The model under review builds one solid part; all positions refer to its coordinate system, in mm. A direction names the side the tool comes from. Round coordinates to 2 decimals unless told otherwise and drop trailing zeros. Write each loop counter-clockwise with the first axis right and the second up, starting at its lowest first coordinate (ties: lowest second). Pieces come first, ordered by that corner, then holes. Notation, with made-up numbers: (-20, -19.5) - (-15, -19.5) arc R28 cw to (-15, -0.5) - close; hole circle Ø3 at (-12, -0.75). An arc over 180 degrees is marked (long way). Write each question's results on one line, items separated by ' | '.
```python
from build123d import *

# Parameters (mm, degrees)
AUFSATZ_LINEAR_AUSTRAGEN1_DEPTH = 145.2
AUFSATZ_LINEAR_AUSTRAGEN2_DEPTH = 145.2
SKIZZE5_R                       = 2.2
SCHNITT_LINEAR_AUSTRAGEN1_DEPTH = 165.848511541
SCHNITT_LINEAR_AUSTRAGEN2_REACH = 166.605
SKIZZE6_W                       = 76.784770152
SKIZZE6_H                       = 124
SKIZZE6_H_2                     = 2.6
SKIZZE7_W                       = 40
SKIZZE7_H                       = 50.4
SCHNITT_LINEAR_AUSTRAGEN3_DEPTH = 166.115329215
SKIZZE8_W                       = 42
SKIZZE8_H                       = 57.4
SCHNITT_LINEAR_AUSTRAGEN4_DEPTH = 3.4


with BuildPart() as part:
    # Skizze1 → Aufsatz-Linear austragen1 (new body)
    with BuildSketch(Plane.XY):
        Polygon((0, 0), (0, 4.329568801), (68.182309499, -23.912468507), (68.182309499, -28.242037309), align=None)
    extrude(amount=AUFSATZ_LINEAR_AUSTRAGEN1_DEPTH)

    # Skizze4 → Aufsatz-Linear austragen2 (add)
    with BuildSketch(Plane.XY.offset(145.2)):
        Polygon((0, 0), (10, -4.142135624), (10, -14.966057627), (0, -10.823922003), align=None)
        Polygon((55.582309499, -23.022946423), (65.582309499, -27.165082046), (65.582309499, -37.989004049), (55.582309499, -33.846868426), align=None)
    extrude(amount=-AUFSATZ_LINEAR_AUSTRAGEN2_DEPTH)

    # Skizze5 → Schnitt-Linear austragen1 (cut, through all)
    with BuildSketch(Plane.XY.offset(145.2)):
        with Locations((5, -7.483028813)):
            Circle(SKIZZE5_R)
        with Locations((60.582309499, -30.505975236)):
            Circle(SKIZZE5_R)
    extrude(amount=-SCHNITT_LINEAR_AUSTRAGEN1_DEPTH, mode=Mode.SUBTRACT)

    # Schnitt-Linear austragen2: up to this face of the body (flat: up to its plane)
    schnitt_linear_austragen2_end = Plane(part.part.faces().sort_by_distance((32.79115475, -13.582541023, 72.6))[0])
    # Skizze6 → Schnitt-Linear austragen2 (cut, up to the picked face)
    with BuildSketch(Plane(origin=(-3.826834324, -9.238795325, 0), x_dir=(0.9238795325112881, -0.3826834323650869, 0), z_dir=(-0.3826834323650869, -0.9238795325112881, 0)), mode=Mode.PRIVATE) as schnitt_linear_austragen2_sk1:
        with Locations((36.735530827, 72.6)):
            Rectangle(SKIZZE6_W, SKIZZE6_H)
    schnitt_linear_austragen2_tool1 = split(extrude(schnitt_linear_austragen2_sk1.sketch, amount=-SCHNITT_LINEAR_AUSTRAGEN2_REACH, mode=Mode.PRIVATE), bisect_by=schnitt_linear_austragen2_end, keep=Keep.BOTH, mode=Mode.PRIVATE)
    # Skizze6 → Schnitt-Linear austragen2 (cut, up to the picked face)
    with BuildSketch(Plane(origin=(-3.826834324, -9.238795325, 0), x_dir=(0.9238795325112881, -0.3826834323650869, 0), z_dir=(-0.3826834323650869, -0.9238795325112881, 0)), mode=Mode.PRIVATE) as schnitt_linear_austragen2_sk2:
        with Locations((36.735530827, 143.9)):
            Rectangle(SKIZZE6_W, SKIZZE6_H_2)
    schnitt_linear_austragen2_tool2 = split(extrude(schnitt_linear_austragen2_sk2.sketch, amount=-SCHNITT_LINEAR_AUSTRAGEN2_REACH, mode=Mode.PRIVATE), bisect_by=schnitt_linear_austragen2_end, keep=Keep.BOTH, mode=Mode.PRIVATE)
    # Skizze6 → Schnitt-Linear austragen2 (cut, up to the picked face)
    with BuildSketch(Plane(origin=(-3.826834324, -9.238795325, 0), x_dir=(0.9238795325112881, -0.3826834323650869, 0), z_dir=(-0.3826834323650869, -0.9238795325112881, 0)), mode=Mode.PRIVATE) as schnitt_linear_austragen2_sk3:
        with Locations((36.735530827, 1.3)):
            Rectangle(SKIZZE6_W, SKIZZE6_H_2)
    schnitt_linear_austragen2_tool3 = split(extrude(schnitt_linear_austragen2_sk3.sketch, amount=-SCHNITT_LINEAR_AUSTRAGEN2_REACH, mode=Mode.PRIVATE), bisect_by=schnitt_linear_austragen2_end, keep=Keep.BOTH, mode=Mode.PRIVATE)
    add(schnitt_linear_austragen2_tool1.solids().sort_by(Axis((30.112371, -23.296874, 72.6), (0.3826834323650869, 0.9238795325112881, 0)))[0], mode=Mode.SUBTRACT)
    add(schnitt_linear_austragen2_tool2.solids().sort_by(Axis((30.112371, -23.296874, 143.9), (0.3826834323650869, 0.9238795325112881, 0)))[0], mode=Mode.SUBTRACT)
    add(schnitt_linear_austragen2_tool3.solids().sort_by(Axis((30.112371, -23.296874, 1.3), (0.3826834323650869, 0.9238795325112881, 0)))[0], mode=Mode.SUBTRACT)

    # Skizze7 → Schnitt-Linear austragen3 (cut, through all)
    with BuildSketch(Plane(origin=(1.530733729, 3.69551813, 0), x_dir=(0.9238795325112881, -0.38268343236508656, 0), z_dir=(0.38268343236508656, 0.9238795325112881, 0))):
        with Locations((35.243145751, -72.6)):
            Rectangle(SKIZZE7_W, SKIZZE7_H)
    extrude(amount=-SCHNITT_LINEAR_AUSTRAGEN3_DEPTH, mode=Mode.SUBTRACT)

    # Skizze8 → Schnitt-Linear austragen4 (cut)
    with BuildSketch(Plane(origin=(0, 0, 0), x_dir=(0.923879532511288, -0.38268343236508684, 0), z_dir=(-0.38268343236508684, -0.923879532511288, 0))):
        with Locations((35.243145751, 75.1)):
            Rectangle(SKIZZE8_W, SKIZZE8_H)
    extrude(amount=-SCHNITT_LINEAR_AUSTRAGEN4_DEPTH, mode=Mode.SUBTRACT)


solid = part.part
```
Q1. We need section B-B (x = 5). State the section outline as (y, z) points.
Evaluation:
outline: (-12.89, 2.6) - (-9.68, 2.6) - (-9.68, 10.6) - (-12.89, 10.6) - close; (-12.89, 134.6) - (-9.68, 134.6) - (-9.68, 142.6) - (-12.89, 142.6) - close; (-5.28, 2.6) - (-2.07, 2.6) - (-2.07, 0) - (2.26, 0) - (2.26, 145.2) - (-2.07, 145.2) - (-2.07, 142.6) - (-5.28, 142.6) - (-5.28, 134.6) - (-2.07, 134.6) - (-2.07, 10.6) - (-5.28, 10.6) - close
Q2. Tool access review of faces 1 (the flat face through (52.603, -19.975, 74.698)), 2 (the flat face through (4, -10, 142.6)), 3 (the flat face through (55.582, -29, 139)), 4 (the flat face through (10, -9, 7)): name each direction out of +Z, -Z, +X, -X, +Y, -Y from which nothing blocks a thin tool from reaching the whole face with its end or side.
Evaluation:
face 1: -X | face 2: +Z, -X, -Y | face 3: +Z, -Z, -X, -Y | face 4: +Z, -Z, -Y
Q3. We need section C-C (z = 20.5). State the section outline as (x, y) points.
Evaluation:
outline: (0, 0) - (68.18, -28.24) - (68.18, -23.91) - (0, 4.33) - close
Q4. For probe 1 along Z at (x, y) = (57.5, -34); probe 2 along Z at (x, y) = (15, -3.5); probe 3 along Y at (x, z) = (5, 7), list the stretches that pass through material, from the lowest coordinate up.
Evaluation:
probe 1: z = 2.6 to 10.6, 134.6 to 142.6 | probe 2: z = 0 to 46.4, 103.8 to 145.2 | probe 3: y = -12.89 to -9.68, -5.28 to 2.26
Q5. Insertion check: P1, Ø5, axis at x = 57.5, z = 90, coming from the +Y side; P2, Ø5, axis at x = 4.5, y = -6.5, coming from the -Z side; P3, Ø3, axis at x = 5, y = -6, coming from the +Z side. Each pin has a flat end and moves straight along its axis. Give the tip position at first contact, or say it passes through.
Evaluation:
P1: stops at y = -18.45 | P2: stops at z = 2.6 | P3: stops at z = 142.6
Q6. The part is to be moulded in two halves that separate along X. For faces 5 (the flat face through (10.89, -0.18, 71.58)), 6 (the flat face through (60.652, -35.947, 6.656)), 7 (the cylindrical face through (62.681, -29.845, 138.656)), say which applies: released by +X, released by -X, zero draft, split by the parting line, or undercut.
Evaluation:
face 5: released by +X | face 6: released by -X | face 7: undercut
Q7. We need section A-A (x = 44). State the section outline as (y, z) points, plus the area to 3 significant figures.
Evaluation:
outline: (-18.23, 0) - (-13.9, 0) - (-13.9, 47.4) - (-14.55, 47.4) - (-14.55, 46.4) - (-18.23, 46.4) - close; (-18.23, 103.8) - (-14.55, 103.8) - (-14.55, 97.8) - (-13.9, 97.8) - (-13.9, 145.2) - (-18.23, 145.2) - close | area: 385 mm^2
